Could you check a few things on this model? Use its own coordinates, in mm. A direction names the side the tool comes from. Round coordinates to 2 decimals unless told otherwise and drop trailing zeros. Loops run counter-clockwise (first coordinate to the right, second up) from the corner with the lowest first, then second, coordinate; pieces in that order, holes last. Notation, with made-up numbers: M -35,-31 L 6,-31 A22 cw 6,-11 Z; hole C 65,-1 d6. An arc over 180 degrees is marked long. Return JSON: item names as keys, results as strings. Group by question number.
```python
from build123d import *

# Parameters (mm, degrees)
F0_W     = 3.81
F0_H     = 17.78
F0_W_2   = 3.802742
F0_H_2   = 9.8044
F1_DEPTH = 2.159
F2_R     = 0.889
F3_DEPTH = 12.192
F4_R     = 1.016
F5_DEPTH = 5.842
F6_W     = 2.159
F6_H     = 6.9596
F7_DEPTH = 19.177


with BuildPart() as f1:
    # F0 (on Top) → F1 (new body)
    with BuildSketch(Plane.XY):
        with BuildLine():
            Line((9.2456, -6.1341), (29.21, -6.1341))
            ThreePointArc((29.21, -6.1341), (31.904077, -5.018177), (33.02, -2.3241))
            Line((33.02, -2.3241), (33.02, 2.3241))
            ThreePointArc((33.02, 2.3241), (31.904077, 5.018177), (29.21, 6.1341))
            Line((29.21, 6.1341), (9.2456, 6.1341))
            Line((9.2456, 6.1341), (5.442858, 6.1341))
            Line((5.442858, 6.1341), (-5.4356, 6.1341))
            Line((-5.4356, 6.1341), (-9.2456, 6.1341))
            Line((-9.2456, 6.1341), (-29.21, 6.1341))
            ThreePointArc((-29.21, 6.1341), (-31.904077, 5.018177), (-33.02, 2.3241))
            Line((-33.02, 2.3241), (-33.02, -2.3241))
            ThreePointArc((-33.02, -2.3241), (-31.904077, -5.018177), (-29.21, -6.1341))
            Line((-29.21, -6.1341), (-9.2456, -6.1341))
            Line((-9.2456, -6.1341), (-5.4356, -6.1341))
            Line((-5.4356, -6.1341), (5.442858, -6.1341))
            Line((5.442858, -6.1341), (9.2456, -6.1341))
        make_face()
        with Locations((-7.3406, 15.0241)):
            Rectangle(F0_W, F0_H)
        with BuildLine():
            Line((5.442858, 23.9141), (9.2456, 23.9141))
            Line((9.2456, 23.9141), (12.0396, 23.9141))
            ThreePointArc((12.0396, 23.9141), (13.835651, 24.658049), (14.5796, 26.4541))
            Line((14.5796, 26.4541), (14.5796, 28.4861))
            ThreePointArc((14.5796, 28.4861), (13.835651, 30.282151), (12.0396, 31.0261))
            Line((12.0396, 31.0261), (-12.0396, 31.0261))
            ThreePointArc((-12.0396, 31.0261), (-13.835651, 30.282151), (-14.5796, 28.4861))
            Line((-14.5796, 28.4861), (-14.5796, 26.4541))
            ThreePointArc((-14.5796, 26.4541), (-13.835651, 24.658049), (-12.0396, 23.9141))
            Line((-12.0396, 23.9141), (-9.2456, 23.9141))
            Line((-9.2456, 23.9141), (-5.4356, 23.9141))
            Line((-5.4356, 23.9141), (0, 23.9141))
            Line((0, 23.9141), (5.442858, 23.9141))
        make_face()
        with Locations((7.344229, 15.0241)):
            Rectangle(F0_W_2, F0_H)
        with Locations((7.344229, -11.0363)):
            Rectangle(F0_W_2, F0_H_2)
        with Locations((-7.3406, -11.0363)):
            Rectangle(F0_W, F0_H_2)
    extrude(amount=F1_DEPTH)

    # F2 (on face) → F3 (join)
    with BuildSketch(Plane.XY.offset(2.159)):
        with Locations((-25.4, 0)):
            Circle(F2_R)
        with Locations((-12.556378, -2.3241)):
            Circle(F2_R)
        with Locations((-12.556378, 2.3241)):
            Circle(F2_R)
        with Locations((25.125987, 0)):
            Circle(F2_R)
        with Locations((12.8016, 2.3368)):
            Circle(F2_R)
        with Locations((12.8016, -2.3368)):
            Circle(F2_R)
    extrude(amount=F3_DEPTH)

    # F4 (on face) → F5 (join)
    with BuildSketch(Plane.XY.offset(2.159)):
        with Locations((-8.74776, 27.4701)):
            Circle(F4_R)
        with Locations((-2.91592, 27.4701)):
            Circle(F4_R)
        with Locations((2.91592, 27.4701)):
            Circle(F4_R)
        with Locations((8.74776, 27.4701)):
            Circle(F4_R)
    extrude(amount=F5_DEPTH)

    # F6 (on face) → F7 (join)
    with BuildSketch(Plane.XY.offset(2.159)):
        with Locations((-7.3406, -11.0363)):
            Rectangle(F6_W, F6_H)
        with Locations((7.347858, -11.0363)):
            Rectangle(F6_W, F6_H)
    extrude(amount=F7_DEPTH)


solid = f1.part
```
1. If we section it at A-A, the plane z = 17.5: Please give me the cut outline in (x, y), then the cut area to 3 significant figures.
2. We'd pull the mould along X, two halves only. Please class faces 1 (the face through (-13.445, -2.285, 8.17)), 2 (the face through (19, 6.134, 1)), 3 (the face through (9.246, -11, 1)), 4 (the face through (-13.82, 30.3, 1.06)): +X half, -X half, draft (parallel to the pull), parting line (faces both ways), or undercut.
3. If we section it at D-D, the plane z = 3.5: Give the number of separate pieces and of enclosed holes in the cut face, then the cut area to 3 significant figures.
4. If we section it at B-B, the plane y = 14.5: Please give me the cut outline in (x, z).
5. I'm going to push flat-ended pins straight in: pin 1 Ø8 at (x, z) = (-17, 11) entering from +Y; pin 2 Ø0.6 at (y, z) = (13, 1.5) entering from +X; pin 3 Ø0.9 at (x, y) = (13, 2.5) entering from +Z; pin 4 Ø10 at (x, z) = (6.5, 2.5) entering from -Y. Where does each tip first touch, or does it pass through?
6. If we section it at C-C, the plane x = -3: Please give me the cut outline in (y, z).
7. On a 3-axis mill with a long thin cutter (end or side, diameter ignored), from which of +Z, -Z, +X, -X, +Y, -Y can I reach the whole of each face in a straight line? I mean faces 5 (the face through (-7, -14.516, 12)), 6 (the face through (9.246, 15, 1)), 7 (the face through (5.443, -11, 1)), 8 (the face through (-19, 6.134, 1)), 9 (the face through (0, 3, 2.159)). Say none if no direction works.
8. I need wall thicknesses on probe 1 along X at (y, z) = (23.5, 1.5); probe 2 along Z at (x, y) = (-24.5, 1.5); probe 3 along X at (y, z) = (2, 6.25). Which ranges of each line are inside material? Lowest first, please.
Geometry results:
{
 "1": {"outline": "M -8.42,-14.52 L -6.26,-14.52 L -6.26,-7.56 L -8.42,-7.56 Z; M 6.27,-14.52 L 8.43,-14.52 L 8.43,-7.56 L 6.27,-7.56 Z", "area": "30.1 mm^2"},
 "2": {"face 1": "undercut", "face 2": "draft", "face 3": "+X half", "face 4": "-X half"},
 "3": {"separate pieces": "12", "enclosed holes": "0", "area": "57.9 mm^2"},
 "4": {"outline": "M -9.25,0 L -5.44,0 L -5.44,2.16 L -9.25,2.16 Z; M 5.44,0 L 9.25,0 L 9.25,2.16 L 5.44,2.16 Z"},
 "5": {"pin 1": "y = 3.09", "pin 2": "x = 9.25", "pin 3": "z = 14.35", "pin 4": "y = -15.94"},
 "6": {"outline": "M -6.13,0 L 6.13,0 L 6.13,2.16 L -6.13,2.16 Z; M 23.91,0 L 31.03,0 L 31.03,2.16 L 28.48,2.16 L 28.48,8 L 26.46,8 L 26.46,2.16 L 23.91,2.16 Z"},
 "7": {"face 5": "+Z, +X, -X, -Y", "face 6": "+Z, -Z, +X", "face 7": "+Z, -Z, -Y", "face 8": "+Z, -Z, -X", "face 9": "+Z"},
 "8": {"probe 1": "-9.25 to -5.44, 5.44 to 9.25", "probe 2": "0 to 2.16", "probe 3": "-13.38 to -11.73, 11.98 to 13.62"}
}
